Read the model definition and answer for the solid it produces. Units are mm, in the model's axes. A direction names the side the tool comes from. Coordinates: 2 decimals unless noted, no trailing zeros. Order: outer loops, then holes, each group sorted by start corner. A loop starts at its lowest first (then second) coordinate and runs counter-clockwise, first axis right, second up. Notation, with made-up numbers: (16.5, -21) -> (60.5, -21) arc R19 cw to (60.5, -5) -> close; hole circle Ø2 at (-2, 19.5). An arc over 180 degrees is marked (long way). Use CSV: the item, a comma, the result in double quotes.
```python
from build123d import *

# Parameters (mm, degrees)
SKETCH1_W           = 60
SKETCH1_H           = 72
BOSS_EXTRUDE1_DEPTH = 18
SKETCH2_W           = 50
SKETCH2_H           = 6.5
CUT_EXTRUDE1_DEPTH  = 81.049984385
SKETCH3_W           = 18
SKETCH3_H           = 30
BOSS_EXTRUDE2_DEPTH = 42
SKETCH4_W           = 7.5
SKETCH4_H           = 20
CUT_EXTRUDE2_DEPTH  = 42.5
SKETCH5_R           = 2.55
CUT_EXTRUDE3_DEPTH  = 35
FILLET1_R           = 5
SKETCH6_R           = 2.55
CUT_EXTRUDE4_DEPTH  = 35


with BuildPart() as part:
    # Sketch1 → Boss-Extrude1 (new body)
    with BuildSketch(Plane.XY):
        Rectangle(SKETCH1_W, SKETCH1_H)
    extrude(amount=BOSS_EXTRUDE1_DEPTH)

    # Sketch2 → Cut-Extrude1 (cut, through all)
    with BuildSketch(Plane(origin=(0, 36, 0), x_dir=(1, 0, 0), z_dir=(0, 1, 0))):
        with Locations((0, -9)):
            Rectangle(SKETCH2_W, SKETCH2_H)
    extrude(amount=-CUT_EXTRUDE1_DEPTH, mode=Mode.SUBTRACT)

    # Sketch3 → Boss-Extrude2 (add)
    with BuildSketch(Plane.ZY.offset(30)):
        with Locations((9, -21)):
            Rectangle(SKETCH3_W, SKETCH3_H)
    boss_extrude2 = extrude(amount=BOSS_EXTRUDE2_DEPTH)

    # Sketch4 → Cut-Extrude2 (cut)
    with BuildSketch(Plane.ZY.offset(72)):
        with Locations((9, -21)):
            Rectangle(SKETCH4_W, SKETCH4_H)
    cut_extrude2 = extrude(amount=-CUT_EXTRUDE2_DEPTH, mode=Mode.SUBTRACT)

    # Sketch5 → Cut-Extrude3 (cut)
    with BuildSketch(Plane.XY.offset(18)):
        with Locations((-64.5, -21)):
            Circle(SKETCH5_R)
        with Locations((-56.2, -21)):
            Circle(SKETCH5_R)
        with Locations((-47.9, -21)):
            Circle(SKETCH5_R)
        with Locations((-39.6, -21)):
            Circle(SKETCH5_R)
    cut_extrude3 = extrude(amount=-CUT_EXTRUDE3_DEPTH, mode=Mode.SUBTRACT)

    # Mirror1: Boss-Extrude2, Cut-Extrude2, Cut-Extrude3 across plane
    add(boss_extrude2.mirror(Plane(origin=(0, 0, 0), x_dir=(0, 0, 1), z_dir=(1, 0, 0))))
    add(cut_extrude2.mirror(Plane(origin=(0, 0, 0), x_dir=(0, 0, 1), z_dir=(1, 0, 0))), mode=Mode.SUBTRACT)
    add(cut_extrude3.mirror(Plane(origin=(0, 0, 0), x_dir=(0, 0, 1), z_dir=(1, 0, 0))), mode=Mode.SUBTRACT)

    # Fillet1
    fillet1_edges = [part.edges().sort_by_distance(p)[0] for p in [
        (-30, -6, 9),
        (-72, -36, 9),
        (-72, -6, 9),
        (-30, 36, 9),
        (30, 36, 9),
        (72, -6, 9),
        (72, -36, 9),
        (30, -6, 9),
    ]]
    fillet(fillet1_edges, radius=FILLET1_R - 0.0001)  # a hair under: the kernel refuses the full size

    # Sketch6 → Cut-Extrude4 (cut)
    with BuildSketch(Plane.XY.offset(18)):
        Circle(SKETCH6_R)
        with Locations((0, 10)):
            Circle(SKETCH6_R)
    extrude(amount=-CUT_EXTRUDE4_DEPTH, mode=Mode.SUBTRACT)


solid = part.part
```
Item 1: Each of these flat-tipped pins is pushed along its axis until it touches: P1, Ø3, axis at y = 2.5, z = 9.5, coming from the -X side; P2, Ø3, axis at x = -44.5, z = 15.5, coming from the +Y side; P3, Ø5, axis at y = 23, z = 9.5, coming from the +X side. Where does it stop, or does it pass through?
Return value:
P1,"stops at x = -30"
P2,"stops at y = -6"
P3,"stops at x = 30"
Item 2: Straight lines are drawn through the part: line 1 along Y through (x, z) = (0, 2); line 2 along Z through (x, y) = (14.5, 3.5); line 3 along X through (y, z) = (4, 6.75). For each, find the intervals that lie inside material, in ascending order.
Return value:
line 1,"y = -36 to -2.55, 2.55 to 7.45, 12.55 to 36"
line 2,"z = 0 to 5.75, 12.25 to 18"
line 3,"x = -30 to -25, 25 to 30"
Item 3: The mould has two halves that part along Z. Classify faces 1 (the flat face through (51, -21, 12.75)), 2 (the flat face through (51, -31, 9)), 3 (the flat face through (-1, -36, 13)): +Z half, -Z half, draft (parallel to the pull), parting line (faces both ways), or undercut.
Return value:
face 1,"undercut"
face 2,"undercut"
face 3,"draft"
Item 4: Find section D-D, the plane x = -64.5. Give the vertices of the cut face in (y, z), then the cut area to 3 significant figures.
Return value:
outline,"(-36, 0) -> (-23.55, 0) -> (-23.55, 5.25) -> (-31, 5.25) -> (-31, 12.75) -> (-23.55, 12.75) -> (-23.55, 18) -> (-36, 18) -> close; (-18.45, 0) -> (-6, 0) -> (-6, 18) -> (-18.45, 18) -> (-18.45, 12.75) -> (-11, 12.75) -> (-11, 5.25) -> (-18.45, 5.25) -> close"
area,"336 mm^2"
Item 5: Find section C-C, the plane x = 7. Give the vertices of the cut face in (y, z), then the cut area to 3 significant figures.
Return value:
outline,"(-36, 0) -> (36, 0) -> (36, 5.75) -> (-36, 5.75) -> close; (-36, 12.25) -> (36, 12.25) -> (36, 18) -> (-36, 18) -> close"
area,"828 mm^2"
Item 6: Find section A-A, the plane y = 22. Give the vertices of the cut face in (x, z), then the cut area to 3 significant figures.
Return value:
outline,"(-30, 0) -> (30, 0) -> (30, 18) -> (-30, 18) -> close; hole (-25, 5.75) -> (25, 5.75) -> (25, 12.25) -> (-25, 12.25) -> close"
area,"755 mm^2"
Item 7: A tool of negligible diameter and unlimited length cuts with its end or side. For faces 4 (the flat face through (29.5, -21, 9)), 5 (the cylindrical face through (-29, 34, 9)), 6 (the flat face through (30, 15, 9)), from which of +Z, -Z, +X, -X, +Y, -Y can it reach the whole face along a straight path? Write none if from no direction.
Return value:
face 4,"+X"
face 5,"+Z, -Z, -X, +Y"
face 6,"+Z, -Z, +X, +Y"
